Here's how the part is built. I have some questions about the finished solid (model axes, mm). A direction names the side the tool comes from. Coordinates: 2 decimals unless noted, no trailing zeros. Loops run counter-clockwise (first coordinate to the right, second up) from the corner with the lowest first, then second, coordinate; pieces in that order, holes last. Notation, with made-up numbers: (55, 71) -> (85, 71) arc R23 cw to (85, 101) -> close; hole circle Ø5 at (-18, -10). An arc over 180 degrees is marked (long way). Answer as a JSON object with one key per item and string values. Group by question number.
1) I want a section at A-A (y = 7.5). Write out the boundary of the cut face in (x, z).
2) I need wall thicknesses on probe 1 along Y at (x, z) = (-10.25, -1.25); probe 2 along Z at (x, y) = (-11.75, 7); probe 3 along Y at (x, z) = (-24.5, 1.25). Which ranges of each line are inside material? Lowest first, please. Write a range as [from, to].
3) I'm going to push flat-ended pins straight in: pin 1 (6 mm diameter, centred on x = -24, y = 8.5, fed in from +Z); pin 2 (2 mm diameter, centred on x = -26, z = 3.5, fed in from -Y); pin 3 (1.5 mm diameter, centred on y = 8.5, z = 2, fed in from +X); pin 4 (1.5 mm diameter, centred on x = -24, y = 7.5, fed in from -Z). Where does each tip first touch, or does it pass through?
4) I want a section at B-B (x = -24.5). Write out the boundary of the cut face in (y, z).
5) I want a section at D-D (x = -9.5). Write out the boundary of the cut face in (y, z), then the cut area to 3 significant figures.
6) If we mould it in two halves opening along X, with no side actions, what happens to faces 1 (the flat face through (-27.272, 7, 1)), 2 (the flat face through (-10.272, 7, 1)), 3 (the cylindrical face through (-13.725, 7.8, 1.413))? For each: +X half, -X half, draft (parallel to the pull), parting line (faces both ways), or undercut.
7) I want a section at C-C (z = 2). Write out the boundary of the cut face in (x, y).
8) Which directions (+Z, -Z, +X, -X, +Y, -Y) give clear straight access to the entire face, cutting with the end or side of a thin tool? Please do faces 4 (the flat face through (-25, 9, -0.066)), 5 (the flat face through (-25, 9, 2.934)), 6 (the flat face through (-15.272, 7, 1)).
```python
from build123d import *

# Parameters (mm, degrees)
SKETCH2_W           = 24
SKETCH2_H           = 20
BOSS_EXTRUDE1_DEPTH = 5
SKETCH3_W           = 5
SKETCH3_H           = 3
BOSS_EXTRUDE2_DEPTH = 5
SKETCH5_R           = 1
CUT_EXTRUDE2_DEPTH  = 3
SKETCH6_R           = 1
CUT_EXTRUDE3_DEPTH  = 3
SKETCH7_R           = 1.5
CUT_EXTRUDE4_DEPTH  = 5


with BuildPart() as part:
    # Sketch2 → Boss-Extrude1 (new body)
    with BuildSketch(Plane(origin=(0, 0, 0), x_dir=(1, 0, 0), z_dir=(0, 1, 0))):
        with Locations((-18.771651872, -1.433503677)):
            Rectangle(SKETCH2_W, SKETCH2_H)
    extrude(amount=BOSS_EXTRUDE1_DEPTH)

    # Sketch3 → Boss-Extrude2 (add)
    with BuildSketch(Plane(origin=(0, 5, 0), x_dir=(1, 0, 0), z_dir=(0, 1, 0))):
        with Locations((-12.771651872, -1.433503677)):
            Rectangle(SKETCH3_W, SKETCH3_H)
        with Locations((-24.771651872, -1.433503677)):
            Rectangle(SKETCH3_W, SKETCH3_H)
    extrude(amount=BOSS_EXTRUDE2_DEPTH)

    # Sketch5 → Cut-Extrude2 (cut)
    with BuildSketch(Plane(origin=(0, 0, -0.066496323), x_dir=(-1, 0, 0), z_dir=(0, 0, -1))):
        with Locations((12.771651872, 7.5)):
            Circle(SKETCH5_R)
    extrude(amount=-CUT_EXTRUDE2_DEPTH, mode=Mode.SUBTRACT)

    # Sketch6 → Cut-Extrude3 (cut)
    with BuildSketch(Plane(origin=(0, 0, -0.066496323), x_dir=(-1, 0, 0), z_dir=(0, 0, -1))):
        with Locations((24.771651872, 7.5)):
            Circle(SKETCH6_R)
    extrude(amount=-CUT_EXTRUDE3_DEPTH, mode=Mode.SUBTRACT)

    # Sketch7 → Cut-Extrude4 (cut)
    with BuildSketch(Plane(origin=(0, 5, 0), x_dir=(1, 0, 0), z_dir=(0, 1, 0))):
        with Locations((-18.771651872, -1.433503677)):
            Circle(SKETCH7_R)
    extrude(amount=-CUT_EXTRUDE4_DEPTH, mode=Mode.SUBTRACT)


solid = part.part
```
Determined:
{
 "1": {"outline": "(-27.27, -0.07) -> (-25.77, -0.07) -> (-25.77, 2.93) -> (-27.27, 2.93) -> close; (-23.77, -0.07) -> (-22.27, -0.07) -> (-22.27, 2.93) -> (-23.77, 2.93) -> close; (-15.27, -0.07) -> (-13.77, -0.07) -> (-13.77, 2.93) -> (-15.27, 2.93) -> close; (-11.77, -0.07) -> (-10.27, -0.07) -> (-10.27, 2.93) -> (-11.77, 2.93) -> close"},
 "2": {"probe 1": "[0, 5]", "probe 2": "[-0.07, 2.93]", "probe 3": "[0, 6.54], [8.46, 10]"},
 "3": {"pin 1": "z = 2.93", "pin 2": "y = 0", "pin 3": "x = -10.27", "pin 4": "z = -0.07"},
 "4": {"outline": "(0, -8.57) -> (5, -8.57) -> (5, -0.07) -> (6.54, -0.07) -> (6.54, 2.93) -> (5, 2.93) -> (5, 11.43) -> (0, 11.43) -> close; (8.46, -0.07) -> (10, -0.07) -> (10, 2.93) -> (8.46, 2.93) -> close"},
 "5": {"outline": "(0, -8.57) -> (5, -8.57) -> (5, 11.43) -> (0, 11.43) -> close", "area": "100 mm^2"},
 "6": {"face 1": "-X half", "face 2": "+X half", "face 3": "undercut"},
 "7": {"outline": "(-30.77, 0) -> (-20.16, 0) -> (-20.16, 5) -> (-22.27, 5) -> (-22.27, 10) -> (-27.27, 10) -> (-27.27, 5) -> (-30.77, 5) -> close; (-17.38, 0) -> (-6.77, 0) -> (-6.77, 5) -> (-10.27, 5) -> (-10.27, 10) -> (-15.27, 10) -> (-15.27, 5) -> (-17.38, 5) -> close; hole circle Ø2 at (-24.77, 7.5); hole circle Ø2 at (-12.77, 7.5)"},
 "8": {"face 4": "-Z, +X, -X, +Y", "face 5": "+Z, +X, -X, +Y", "face 6": "+Z, -Z, +Y"}
}
